from build123d import *

# Parameters (mm, degrees)
SKETCH010_W  = 118
SKETCH010_H  = 26
SKETCH010_R  = 3.1
PAD010_DEPTH = 5
SKETCH011_W  = 118
SKETCH011_H  = 4
PAD011_DEPTH = 16
FILLET005_R  = 4.9
FILLET006_R  = 3.9


with BuildPart() as part:
    # Sketch010 → Pad010 (new body)
    with BuildSketch(Plane.XY):
        with Locations((0, 5)):
            Rectangle(SKETCH010_W, SKETCH010_H)
        with Locations((4.1, 11.1)):
            Circle(SKETCH010_R, mode=Mode.SUBTRACT)
        with Locations((36.3, 11.1)):
            Circle(SKETCH010_R, mode=Mode.SUBTRACT)
    extrude(amount=PAD010_DEPTH)

    # Sketch011 (on Face8 of Pad010) → Pad011 (join)
    with BuildSketch(Plane.XY.offset(5)):
        with Locations((0, -6)):
            Rectangle(SKETCH011_W, SKETCH011_H)
    extrude(amount=PAD011_DEPTH)

    # Fillet005
    fillet005_edges = [part.edges().sort_by_distance(p)[0] for p in [
        (0, -8, 0),
    ]]
    fillet(fillet005_edges, radius=FILLET005_R)

    # Fillet006
    fillet006_edges = [part.edges().sort_by_distance(p)[0] for p in [
        (-59, -6.564823, 1.435177),
        (59, -6.564823, 1.435177),
    ]]
    fillet(fillet006_edges, radius=FILLET006_R)


with BuildPart() as part_1:
    # Body009 placement: moved
    add(part.part.moved(Location((272, 160, 0))))


solid = part_1.part
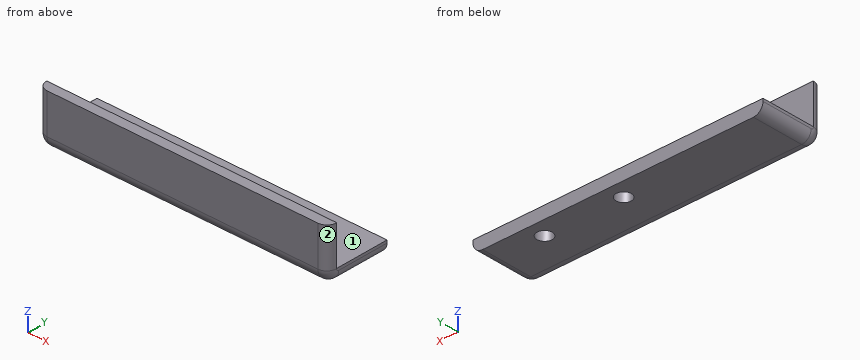
Geometry check sheet. Reference: the model listing, model coordinates, mm. Face numbers are marked on the shaded views. A direction names the side the tool comes from. Give positions to 0.01 mm unless a question says otherwise; leave off trailing zeros. Order: outer loops, then holes, each group sorted by start corner. A loop starts at its lowest first (then second) coordinate and runs counter-clockwise, first axis right, second up. Notation, with made-up numbers: (52, -3.5) - (75, -3.5) arc R11 ccw to (75, 5.5) - close; hole circle Ø2 at (58.5, 76.5). An arc over 180 degrees is marked (long way). Answer as a JSON object with one key per item and string values.
(1) Cross-section at C-C (x = 232.5). Record the cut outline in (y, z).
Report:
{"outline": "(152, 4.9) arc R4.9 ccw to (156.9, 0) - (178, 0) - (178, 5) - (156, 5) - (156, 21) - (152, 21) - close"}
(2) Cross-section at D-D (y = 161.25). Record the cut outline in (x, z), then the cut area to 3 significant figures.
Report:
{"outline": "(213, 3.9) arc R3.9 ccw to (216.9, 0) - (327.1, 0) arc R3.9 ccw to (331, 3.9) - (331, 5) - (213, 5) - close", "area": "583 mm^2"}
(3) Material ranges on line 1 (Z direction, x = 239.5, y = 170.5); line 2 (Y direction, x = 315.5, z = 10.75); line 3 (X direction, y = 163.25, z = 3.75), recorded low to high.
Report:
{"line 1": "0 to 5", "line 2": "152 to 156", "line 3": "213 to 331"}
(4) Cross-section at B-B (y = 171.1). Record the cut outline in (x, z), then the cut area to 3 significant figures.
Report:
{"outline": "(213, 3.9) arc R3.9 ccw to (216.9, 0) - (273, 0) - (273, 5) - (213, 5) - close; (279.2, 0) - (305.2, 0) - (305.2, 5) - (279.2, 5) - close; (311.4, 0) - (327.1, 0) arc R3.9 ccw to (331, 3.9) - (331, 5) - (311.4, 5) - close", "area": "521 mm^2"}
(5) Tool access check on the marked faces 1 and 2. Record the directions out of +Z, -Z, +X, -X, +Y, -Y that give a thin tool (end or side, any length) a straight path to the whole face; none if there is none.
Report:
{"face 1": "+Z, +X, -X, +Y", "face 2": "+Z, -Z, +X, -Y"}
(6) Depth check by flat-ended pin: pin 1 Ø1 at (x, y) = (269.5, 169) entering from +Z; pin 2 Ø5 at (x, z) = (294, 16) entering from +Y. Enter the tip coordinate at first touch or a pass-through.
Report:
{"pin 1": "z = 5", "pin 2": "y = 156"}
(7) Cross-section at A-A (x = 308.3). Record the cut outline in (y, z), then the cut area to 3 significant figures.
Report:
{"outline": "(152, 4.9) arc R4.9 ccw to (156.9, 0) - (168, 0) - (168, 5) - (156, 5) - (156, 21) - (152, 21) - close; (174.2, 0) - (178, 0) - (178, 5) - (174.2, 5) - close", "area": "158 mm^2"}
